Could you check a few things on this drawing? It's one solid part, dimensions in mm from its lowest x, y, z. Coordinates: 2 decimals unless noted, no trailing zeros. Write each loop counter-clockwise with the first axis right and the second up, starting at its lowest first coordinate (ties: lowest second). Pieces come first, ordered by that corner, then holes. Notation, with made-up numbers: M -37.75,66.5 L -30.75,66.5 A19 ccw -30.75,93.5 Z; hole C 10,75 d1. An arc over 180 degrees is marked long. Use a Markdown table: item, result.
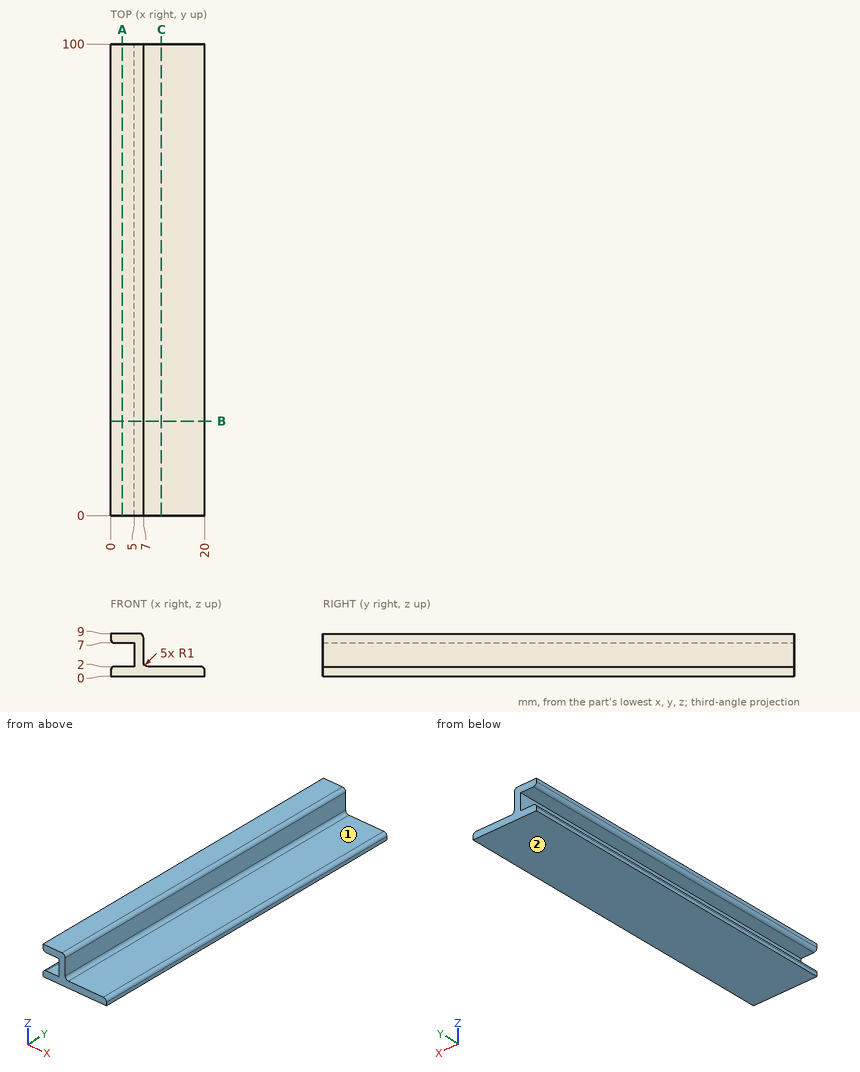
1. Suppose I cut it at A-A on x = 2.5. Write out the boundary of the cut face in (y, z).
Answers follow:
| item | result |
|---|---|
| outline | M 0,0 L 100,0 L 100,2 L 0,2 Z; M 0,7 L 100,7 L 100,9 L 0,9 Z |
2. We'd pull the mould along Z, two halves only. Please class the marked faces 1 and 2: +Z half, -Z half, draft (parallel to the pull), parting line (faces both ways), or undercut.
Answers follow:
| item | result |
|---|---|
| face 1 | +Z half |
| face 2 | -Z half |
3. Suppose I cut it at B-B on y = 20. Write out the boundary of the cut face in (x, z), and give its area (3 significant figures).
Answers follow:
| item | result |
|---|---|
| outline | M 0,0 L 20,0 L 20,1 A1 ccw 19,2 L 8,2 A1 cw 7,3 L 7,8 A1 ccw 6,9 L 0,9 L 0,8 A1 ccw 1,7 L 5,7 L 5,2 L 1,2 A1 ccw 0,1 Z |
| area | 63.4 mm2 |
4. Will these pins go through, and if not, where does the flat tip stop? pin 1 Ø1 at (x, y) = (16, 43.5) entering from +Z; pin 2 Ø2.5 at (y, z) = (63, 4.5) entering from +X; pin 3 Ø4 at (y, z) = (44, 4.5) entering from -X.
Answers follow:
| item | result |
|---|---|
| pin 1 | stops at z = 2 |
| pin 2 | stops at x = 7 |
| pin 3 | stops at x = 5 |
5. Suppose I cut it at C-C on x = 10.75. Write out the boundary of the cut face in (y, z), and give its area (3 significant figures).
Answers follow:
| item | result |
|---|---|
| outline | M 0,0 L 100,0 L 100,2 L 0,2 Z |
| area | 200 mm2 |
6. I need wall thicknesses on probe 1 along Z at (x, y) = (3, 77.5); probe 2 along Z at (x, y) = (15.25, 6.5); probe 3 along X at (y, z) = (24.5, 8). Which ranges of each line are inside material? Lowest first, please.
Answers follow:
| item | result |
|---|---|
| probe 1 | z = 0 to 2, 7 to 9 |
| probe 2 | z = 0 to 2 |
| probe 3 | x = 0 to 7 |
